```python
from build123d import *

# Parameters (mm, degrees)
BOSS_EXTRUDE1_DEPTH = 12


with BuildPart() as part:
    # Sketch1 → Boss-Extrude1 (new body)
    with BuildSketch(Plane.XY):
        with BuildLine():
            Line((230.263882669, 423.104693141), (230.263882669, -376.895306859))
            Line((230.263882669, -376.895306859), (-219.736117331, -376.895306859))
            Line((-219.736117331, -376.895306859), (-119.736117331, 423.104693141))
            Line((-119.736117331, 423.104693141), (-119.736117331, 1223.104693141))
            Line((-119.736117331, 1223.104693141), (-69.736117331, 1223.104693141))
            Line((-69.736117331, 1223.104693141), (-69.736117331, 1218.104693141))
            Line((-69.736117331, 1218.104693141), (-69.736117331, 1214.38315411))
            ThreePointArc((-69.736117331, 1214.38315411), (-70.233173605, 1210.607636866), (-66.457656361, 1211.104693141))
            Line((-66.457656361, 1211.104693141), (-23.0145783, 1211.104693141))
            ThreePointArc((-23.0145783, 1211.104693141), (-19.239061056, 1210.607636866), (-19.736117331, 1214.38315411))
            Line((-19.736117331, 1214.38315411), (-19.736117331, 1218.104693141))
            Line((-19.736117331, 1218.104693141), (-19.736117331, 1223.104693141))
            Line((-19.736117331, 1223.104693141), (30.263882669, 1223.104693141))
            Line((30.263882669, 1223.104693141), (30.263882669, 1218.104693141))
            Line((30.263882669, 1218.104693141), (30.263882669, 1214.38315411))
            ThreePointArc((30.263882669, 1214.38315411), (29.766826395, 1210.607636866), (33.542343639, 1211.104693141))
            Line((33.542343639, 1211.104693141), (76.9854217, 1211.104693141))
            ThreePointArc((76.9854217, 1211.104693141), (80.760938944, 1210.607636866), (80.263882669, 1214.38315411))
            Line((80.263882669, 1214.38315411), (80.263882669, 1218.104693141))
            Line((80.263882669, 1218.104693141), (80.263882669, 1223.104693141))
            Line((80.263882669, 1223.104693141), (130.263882669, 1223.104693141))
            Line((130.263882669, 1223.104693141), (130.263882669, 1218.104693141))
            Line((130.263882669, 1218.104693141), (130.263882669, 1214.38315411))
            ThreePointArc((130.263882669, 1214.38315411), (129.766826395, 1210.607636866), (133.542343639, 1211.104693141))
            Line((133.542343639, 1211.104693141), (176.9854217, 1211.104693141))
            ThreePointArc((176.9854217, 1211.104693141), (180.760938944, 1210.607636866), (180.263882669, 1214.38315411))
            Line((180.263882669, 1214.38315411), (180.263882669, 1223.104693141))
            Line((180.263882669, 1223.104693141), (230.263882669, 1223.104693141))
            Line((230.263882669, 1223.104693141), (230.263882669, 423.104693141))
        make_face()
        with BuildLine():
            Line((-66.457391449, 862.104693141), (-23.014843212, 862.104693141))
            ThreePointArc((-23.014843212, 862.104693141), (-19.239248423, 862.602395721), (-19.736117331, 858.82669113))
            Line((-19.736117331, 858.82669113), (-19.736117331, 853.382695152))
            ThreePointArc((-19.736117331, 853.382695152), (-19.239248423, 849.606990561), (-23.014843212, 850.104693141))
            Line((-23.014843212, 850.104693141), (-66.457391449, 850.104693141))
            ThreePointArc((-66.457391449, 850.104693141), (-70.232986238, 849.606990561), (-69.736117331, 853.382695152))
            Line((-69.736117331, 853.382695152), (-69.736117331, 858.82669113))
            ThreePointArc((-69.736117331, 858.82669113), (-70.232986238, 862.602395721), (-66.457391449, 862.104693141))
        make_face(mode=Mode.SUBTRACT)
        with BuildLine():
            Line((33.542343639, 862.104693141), (76.9854217, 862.104693141))
            ThreePointArc((76.9854217, 862.104693141), (80.760938944, 862.601749416), (80.263882669, 858.826232172))
            Line((80.263882669, 858.826232172), (80.263882669, 853.38315411))
            ThreePointArc((80.263882669, 853.38315411), (80.760938944, 849.607636866), (76.9854217, 850.104693141))
            Line((76.9854217, 850.104693141), (33.542343639, 850.104693141))
            ThreePointArc((33.542343639, 850.104693141), (29.766826395, 849.607636866), (30.263882669, 853.38315411))
            Line((30.263882669, 853.38315411), (30.263882669, 858.826232172))
            ThreePointArc((30.263882669, 858.826232172), (29.766826395, 862.601749416), (33.542343639, 862.104693141))
        make_face(mode=Mode.SUBTRACT)
        with BuildLine():
            Line((130.263882669, 858.823377008), (130.263882669, 853.386009273))
            ThreePointArc((130.263882669, 853.386009273), (129.759845585, 849.609661156), (133.537384707, 850.104693141))
            Line((133.537384707, 850.104693141), (176.990380631, 850.104693141))
            ThreePointArc((176.990380631, 850.104693141), (180.767919754, 849.609661156), (180.263882669, 853.386009273))
            Line((180.263882669, 853.386009273), (180.263882669, 858.823377008))
            ThreePointArc((180.263882669, 858.823377008), (180.767919754, 862.599725126), (176.990380631, 862.104693141))
            Line((176.990380631, 862.104693141), (133.537384707, 862.104693141))
            ThreePointArc((133.537384707, 862.104693141), (129.759845585, 862.599725126), (130.263882669, 858.823377008))
        make_face(mode=Mode.SUBTRACT)
        with BuildLine():
            Line((-66.459371529, -326.895306859), (-23.012863132, -326.895306859))
            ThreePointArc((-23.012863132, -326.895306859), (-19.237850179, -327.388185527), (-19.736117331, -323.613880024))
            Line((-19.736117331, -323.613880024), (-19.736117331, -318.176733694))
            ThreePointArc((-19.736117331, -318.176733694), (-19.237850179, -314.402428191), (-23.012863132, -314.895306859))
            Line((-23.012863132, -314.895306859), (-66.459371529, -314.895306859))
            ThreePointArc((-66.459371529, -314.895306859), (-70.234384482, -314.402428191), (-69.736117331, -318.176733694))
            Line((-69.736117331, -318.176733694), (-69.736117331, -323.613880024))
            ThreePointArc((-69.736117331, -323.613880024), (-70.234384482, -327.388185527), (-66.459371529, -326.895306859))
        make_face(mode=Mode.SUBTRACT)
        with BuildLine():
            Line((33.542343639, -326.895306859), (76.9854217, -326.895306859))
            ThreePointArc((76.9854217, -326.895306859), (80.760938944, -327.392363134), (80.263882669, -323.61684589))
            Line((80.263882669, -323.61684589), (80.263882669, -318.173767828))
            ThreePointArc((80.263882669, -318.173767828), (80.760938944, -314.398250584), (76.9854217, -314.895306859))
            Line((76.9854217, -314.895306859), (33.542343639, -314.895306859))
            ThreePointArc((33.542343639, -314.895306859), (29.766826395, -314.398250584), (30.263882669, -318.173767828))
            Line((30.263882669, -318.173767828), (30.263882669, -323.61684589))
            ThreePointArc((30.263882669, -323.61684589), (29.766826395, -327.392363134), (33.542343639, -326.895306859))
        make_face(mode=Mode.SUBTRACT)
        with BuildLine():
            Line((133.541000442, -326.895306859), (176.986764897, -326.895306859))
            ThreePointArc((176.986764897, -326.895306859), (180.762830308, -327.39181479), (180.263882669, -323.616070974))
            Line((180.263882669, -323.616070974), (180.263882669, -318.174542745))
            ThreePointArc((180.263882669, -318.174542745), (180.762830308, -314.398798928), (176.986764897, -314.895306859))
            Line((176.986764897, -314.895306859), (133.541000442, -314.895306859))
            ThreePointArc((133.541000442, -314.895306859), (129.764935031, -314.398798928), (130.263882669, -318.174542745))
            Line((130.263882669, -318.174542745), (130.263882669, -323.616070974))
            ThreePointArc((130.263882669, -323.616070974), (129.764935031, -327.39181479), (133.541000442, -326.895306859))
        make_face(mode=Mode.SUBTRACT)
        with BuildLine():
            Line((171.542343639, 8.166055965), (176.9854217, 8.166055965))
            ThreePointArc((176.9854217, 8.166055965), (180.760938944, 8.66311224), (180.263882669, 4.887594996))
            Line((180.263882669, 4.887594996), (180.263882669, -38.555483066))
            ThreePointArc((180.263882669, -38.555483066), (180.760938944, -42.33100031), (176.9854217, -41.833944035))
            Line((176.9854217, -41.833944035), (171.542343639, -41.833944035))
            ThreePointArc((171.542343639, -41.833944035), (167.766826395, -42.33100031), (168.263882669, -38.555483066))
            Line((168.263882669, -38.555483066), (168.263882669, 4.887594996))
            ThreePointArc((168.263882669, 4.887594996), (167.766826395, 8.66311224), (171.542343639, 8.166055965))
        make_face(mode=Mode.SUBTRACT)
        with BuildLine():
            Line((168.263882669, -95.112405004), (168.263882669, -138.555483066))
            ThreePointArc((168.263882669, -138.555483066), (167.766826395, -142.33100031), (171.542343639, -141.833944035))
            Line((171.542343639, -141.833944035), (176.9854217, -141.833944035))
            ThreePointArc((176.9854217, -141.833944035), (180.760938944, -142.33100031), (180.263882669, -138.555483066))
            Line((180.263882669, -138.555483066), (180.263882669, -95.112405004))
            ThreePointArc((180.263882669, -95.112405004), (180.760938944, -91.33688776), (176.9854217, -91.833944035))
            Line((176.9854217, -91.833944035), (171.542343639, -91.833944035))
            ThreePointArc((171.542343639, -91.833944035), (167.766826395, -91.33688776), (168.263882669, -95.112405004))
        make_face(mode=Mode.SUBTRACT)
        with BuildLine():
            Line((171.542343639, -191.833944035), (176.9854217, -191.833944035))
            ThreePointArc((176.9854217, -191.833944035), (180.760938944, -191.33688776), (180.263882669, -195.112405004))
            Line((180.263882669, -195.112405004), (180.263882669, -238.555483066))
            ThreePointArc((180.263882669, -238.555483066), (180.760938944, -242.33100031), (176.9854217, -241.833944035))
            Line((176.9854217, -241.833944035), (171.542343639, -241.833944035))
            ThreePointArc((171.542343639, -241.833944035), (167.766826395, -242.33100031), (168.263882669, -238.555483066))
            Line((168.263882669, -238.555483066), (168.263882669, -195.112405004))
            ThreePointArc((168.263882669, -195.112405004), (167.766826395, -191.33688776), (171.542343639, -191.833944035))
        make_face(mode=Mode.SUBTRACT)
        with BuildLine():
            Line((168.263882669, 730.321791286), (168.263882669, 773.764869348))
            ThreePointArc((168.263882669, 773.764869348), (167.766826395, 777.540386592), (171.542343639, 777.043330317))
            Line((171.542343639, 777.043330317), (176.9854217, 777.043330317))
            ThreePointArc((176.9854217, 777.043330317), (180.760938944, 777.540386592), (180.263882669, 773.764869348))
            Line((180.263882669, 773.764869348), (180.263882669, 730.321791286))
            ThreePointArc((180.263882669, 730.321791286), (180.760938944, 726.546274042), (176.9854217, 727.043330317))
            Line((176.9854217, 727.043330317), (171.542343639, 727.043330317))
            ThreePointArc((171.542343639, 727.043330317), (167.766826395, 726.546274042), (168.263882669, 730.321791286))
        make_face(mode=Mode.SUBTRACT)
        with BuildLine():
            Line((171.542343639, 627.043330317), (176.9854217, 627.043330317))
            ThreePointArc((176.9854217, 627.043330317), (180.760938944, 626.546274042), (180.263882669, 630.321791286))
            Line((180.263882669, 630.321791286), (180.263882669, 673.764869348))
            ThreePointArc((180.263882669, 673.764869348), (180.760938944, 677.540386592), (176.9854217, 677.043330317))
            Line((176.9854217, 677.043330317), (171.542343639, 677.043330317))
            ThreePointArc((171.542343639, 677.043330317), (167.766826395, 677.540386592), (168.263882669, 673.764869348))
            Line((168.263882669, 673.764869348), (168.263882669, 630.321791286))
            ThreePointArc((168.263882669, 630.321791286), (167.766826395, 626.546274042), (171.542343639, 627.043330317))
        make_face(mode=Mode.SUBTRACT)
        with BuildLine():
            Line((168.263882669, 530.321791286), (168.263882669, 573.764869348))
            ThreePointArc((168.263882669, 573.764869348), (167.766826395, 577.540386592), (171.542343639, 577.043330317))
            Line((171.542343639, 577.043330317), (176.9854217, 577.043330317))
            ThreePointArc((176.9854217, 577.043330317), (180.760938944, 577.540386592), (180.263882669, 573.764869348))
            Line((180.263882669, 573.764869348), (180.263882669, 530.321791286))
            ThreePointArc((180.263882669, 530.321791286), (180.760938944, 526.546274042), (176.9854217, 527.043330317))
            Line((176.9854217, 527.043330317), (171.542343639, 527.043330317))
            ThreePointArc((171.542343639, 527.043330317), (167.766826395, 526.546274042), (168.263882669, 530.321791286))
        make_face(mode=Mode.SUBTRACT)
    extrude(amount=BOSS_EXTRUDE1_DEPTH)


solid = part.part
```
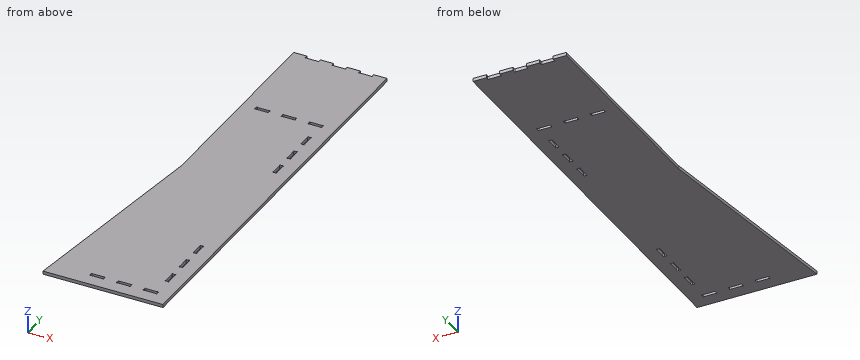
Build history of the part. All positions in model axes, mm. Round coordinates to 2 decimals unless told otherwise and drop trailing zeros. Loops run counter-clockwise (first coordinate to the right, second up) from the corner with the lowest first, then second, coordinate; pieces in that order, holes last. Notation, with made-up numbers: M -3.75,-26.75 L 36.25,-26.75 A30 ccw 36.25,7.25 Z; hole C 19.5,53 d7. An arc over 180 degrees is marked long. Answer as CSV lines item,"result".
1. Cut at A-A on y = 552. Write the cut outline in (x, z), then the cut area to 3 significant figures.
Resolved:
outline,"M -119.74,0 L 168.26,0 L 168.26,12 L -119.74,12 Z; M 180.26,0 L 230.26,0 L 230.26,12 L 180.26,12 Z"
area,"4,060 mm²"
2. Cut at B-B on y = 1032. Write the cut outline in (x, z), then the cut area to 3 significant figures.
Resolved:
outline,"M -119.74,0 L 230.26,0 L 230.26,12 L -119.74,12 Z"
area,"4,200 mm²"
3. Cut at C-C on z = 3. Count the separate pieces of the cut face and the enclosed holes in it, then the cut area to 3 significant figures.
Resolved:
separate pieces,"1"
enclosed holes,"12"
area,"591,000 mm²"
4. Wall check: probe 1 along Y at (x, z) = (142.5, 10.5); probe 2 along Y at (x, z) = (80, 2.75); probe 3 along Y at (x, z) = (-19, 5). Give the ranges that are in metal, low to high. Write a range as [from, to].
Resolved:
probe 1,"y = [-376.9, -326.9], [-314.9, 850.1], [862.1, 1211.1]"
probe 2,"y = [-376.9, -327.91], [-313.89, 849.09], [863.11, 1210.09]"
probe 3,"y = [-376.9, -327.11], [-324.27, -317.52], [-314.68, 849.89], [852.72, 859.49], [862.32, 1210.89], [1213.72, 1223.1]"
5. Cut at D-D on y = 328.5. Write the cut outline in (x, z), then the cut area to 3 significant figures.
Resolved:
outline,"M -131.56,0 L 230.26,0 L 230.26,12 L -131.56,12 Z"
area,"4,340 mm²"
6. Flat gauge pins, fed straight in: P1, Ø2.5, axis at x = 173.5, z = 6, coming from the +Y side; P2, Ø3, axis at y = 404, z = 9, coming from the -X side; P3, Ø5, axis at y = 935, z = 11, coming from the -X side. Where does each tip first touch, or does it go through?
Resolved:
P1,"stops at y = 1211.1"
P2,"stops at x = -122.31"
P3,"stops at x = -119.74"
